Verification items for the finished model (mm, model axes). Give positions to 0.01 mm unless a question says otherwise; leave off trailing zeros. Order: outer loops, then holes, each group sorted by start corner. A loop starts at its lowest first (then second) coordinate and runs counter-clockwise, first axis right, second up. Notation, with made-up numbers: (62.25, 49.25) - (114.25, 49.25) arc R10 ccw to (114.25, 65.25) - close; hole circle Ø3 at (86.25, -34.5). An arc over 180 degrees is marked (long way). Answer as a JSON object with one key per item and string values. Group by question number.
(1) Section check A-A (z = -312). Record the boundary of the cut face in (x, y), then the cut area to 4 significant figures.
(2) Depth check by flat-ended pin: pin 1 Ø2.5 at (y, z) = (2, -197) entering from +X; pin 2 Ø1.5 at (y, z) = (1.5, -390.5) entering from +X; pin 3 Ø1.5 at (x, y) = (-41, 2) entering from -Z. Enter the tip coordinate at first touch or a pass-through.
(3) Section check B-B (y = 3.5). Count the separate pieces of the cut face and the enclosed holes in it, then the cut area to 3 significant figures.
(4) Section check C-C (x = -154). Record the boundary of the cut face in (y, z), then the cut area to 3 significant figures.
(5) Thickness scan on line 1 (Z direction, x = -295, y = 1.35) (1 decimal); line 2 (X direction, y = 4.1, z = -188) (3 decimals); line 3 (X direction, y = 1.9, z = -66.5). Record the ranges inside material, lowest first.
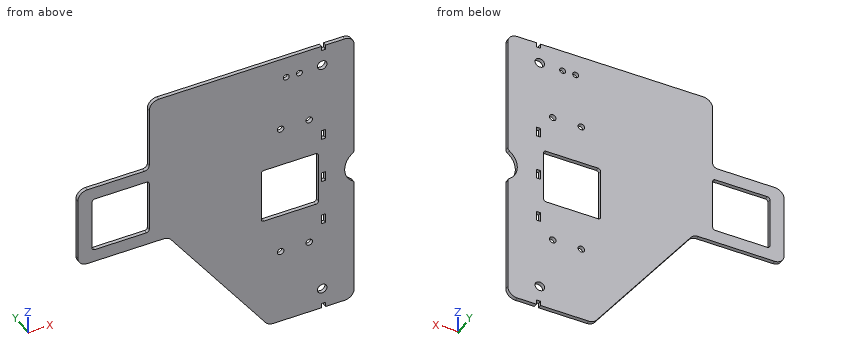
Autodesk Inventor part; units mm, degrees
ref_plane "YZ Plane" through (0, 0, 0) normal (1, 0, 0) x (0, 1, 0)
ref_plane "XZ Plane" through (0, 0, 0) normal (0, 1, 0) x (-1, 0, 0)
ref_plane "XY Plane" through (0, 0, 0) normal (0, 0, 1) x (1, 0, 0)
sketch "Boceto1" plane through (0, 0, 0) normal (0, 1, 0) x (-1, 0, 0)
  line L0 (0, 0) -> (273.05, 0)
  line L1 (273.05, 0) -> (273.05, -101.6)
  line L2 (273.05, -101.6) -> (368.3, -101.6)
  line L3 (368.3, -101.6) -> (368.3, -212.725)
  line L4 (0, 0) -> (0, -393.7)
  line L5 (0, -393.7) -> (114.3, -393.7)
  line L6 (368.3, -212.725) -> (247.65, -212.725)
  line L7 (247.65, -212.725) -> (114.3, -393.7)
  dimension "d0" = 273.05
  dimension "d1" = 101.6
  dimension "d2" = 95.25
  dimension "d3" = 111.125
  dimension "d4" = 393.7
  dimension "d50" = 114.3
  dimension "d51" = 133.35
extrude "Extrusión1" add sketch "Boceto1" along normal blind 5
fillet "Empalme1" radius 12.7 7 edges at (-368.3, 2.5, -101.6) (-273.05, 2.5, 0) (-368.3, 2.5, -212.725) (-247.65, 2.5, -212.725) (-114.3, 2.5, -393.7) (0, 2.5, -393.7) (0, 2.5, 0)
fillet "Empalme2" radius 6.35 1 edges at (-273.05, 2.5, -101.6)
sketch "Boceto2" plane through (0, 5, 0) normal (0, 1, 0) x (1, 0, 0)
  line L0 (-349.25, 119.0625) -> (-273.05, 119.0625)
  line L1 (-273.05, 119.0625) -> (-273.05, 195.2625)
  line L2 (-273.05, 195.2625) -> (-349.25, 195.2625)
  line L3 (-349.25, 195.2625) -> (-349.25, 119.0625)
  line L4 (-368.3, 200.025) -> (-368.3, 114.3)
  line L5 (-254.0674, 212.725) -> (-355.6, 212.725)
  line L6 (-355.6, 101.6) -> (-279.4, 101.6)
  line L7 (-260.35, 0) -> (-12.7, 0)
  line L8 (-43.6563, 0) -> (-38.1, 0)
  line L9 (-38.1, 0) -> (-38.1, 6.35)
  line L10 (-38.1, 6.35) -> (-43.6562, 6.35)
  line L11 (-43.6562, 6.35) -> (-43.6563, 0)
  line L12 (-12.7, 393.7) -> (-107.8826, 393.7)
  line L13 (0, 12.7) -> (0, 381)
  circle A0 centre (-98.0281, 104.775) radius 4.3656
  circle A1 centre (-59.9281, 104.775) radius 4.3656
  circle A2 centre (-98.0281, 288.925) radius 4.3656
  circle A3 centre (-59.9281, 288.925) radius 4.3656
  line L14 (-123.825, 158.75) -> (-47.625, 158.75)
  line L15 (-47.625, 158.75) -> (-47.625, 234.95)
  line L16 (-47.625, 234.95) -> (-123.825, 234.95)
  line L17 (-123.825, 234.95) -> (-123.825, 158.75)
  circle A4 centre (-42.6641, 365.125) radius 6.35
  circle A5 centre (-42.6641, 28.575) radius 6.35
  line L18 (-107.8826, 393.7) -> (-12.7, 393.7)
  line L19 (-43.6563, 393.7) -> (-38.1, 393.7)
  line L20 (-38.1, 393.7) -> (-38.1, 387.35)
  line L21 (-38.1, 387.35) -> (-43.6563, 387.35)
  line L22 (-43.6563, 387.35) -> (-43.6563, 393.7)
  line L23 (-43.6563, 127) -> (-38.1, 127)
  line L24 (-38.1, 127) -> (-38.1, 140.0969)
  line L25 (-38.1, 140.0969) -> (-43.6563, 140.0969)
  line L26 (-43.6563, 140.0969) -> (-43.6563, 127)
  line L27 (-43.6563, 190.5) -> (-38.1, 190.5)
  line L28 (-38.1, 190.5) -> (-38.1, 203.5969)
  line L29 (-38.1, 203.5969) -> (-43.6563, 203.5969)
  line L30 (-43.6563, 203.5969) -> (-43.6563, 190.5)
  line L31 (-43.6563, 254) -> (-38.1, 254)
  line L32 (-38.1, 254) -> (-38.1, 267.0969)
  line L33 (-38.1, 267.0969) -> (-43.6563, 267.0969)
  line L34 (-43.6563, 267.0969) -> (-43.6563, 254)
  circle A6 centre (-73.025, 29.3688) radius 3.9687
  circle A7 centre (-90.4875, 29.3688) radius 3.9688
  point P0 (0, 0)
  dimension "d11" = 76.2
  dimension "d17" = 17.4625
  dimension "d18" = 19.05
  dimension "d19" = 76.2
  dimension "d20" = 5.5563
  dimension "d22" = 6.35
  dimension "d24" = 38.1
  dimension "d27" = 8.7312
  dimension "d38" = 76.2
  dimension "d39" = 76.2
  dimension "d40" = 158.75
  dimension "d42" = 12.7
  dimension "d43" = 28.575
  dimension "d44" = 42.6641
  dimension "d47" = 12.7
  dimension "d52" = 38.1
  dimension "d53" = 5.5563
  dimension "d54" = 6.35
  dimension "d55" = 47.625
  dimension "d56" = 8.7312
  dimension "d57" = 98.0281
  dimension "d58" = 38.1
  dimension "d59" = 53.975
  dimension "d60" = 53.975
  dimension "d61" = 184.15
  dimension "d62" = 184.15
  dimension "d63" = 38.1
  dimension "d64" = 8.7312
  dimension "d65" = 8.7312
  dimension "d66" = 98.0281
  dimension "d67" = 42.6641
  dimension "d68" = 28.575
  dimension "d69" = 5.5563
  dimension "d70" = 5.5563
  dimension "d71" = 5.5563
  dimension "d72" = 13.0969
  dimension "d73" = 13.0969
  dimension "d74" = 13.0969
  dimension "d75" = 38.1
  dimension "d80" = 63.5
  dimension "d81" = 63.5
  dimension "d82" = 127
  dimension "d92" = 7.9375
  dimension "d93" = 7.9375
  dimension "d94" = 25.4
  dimension "d96" = 25.4
  dimension "d97" = 25.4
  dimension "d98" = 25.4
extrude "Extrusión2" cut sketch "Boceto2" against normal up to next
fillet "Empalme3" radius 3.5719 8 edges at (-349.25, 2.5, -119.0625) (-123.825, 2.5, -158.75) (-349.25, 2.5, -195.2625) (-123.825, 2.5, -234.95) (-273.05, 2.5, -195.2625) (-47.625, 2.5, -234.95) (-273.05, 2.5, -119.0625) (-47.625, 2.5, -158.75)
sketch "Boceto3" plane through (0, 5, 0) normal (0, 1, 0) x (1, 0, 0)
  line L0 (0, 12.7) -> (0, 381)
  line L1 (0, 381) -> (0, 12.7)
  line L2 (0, 196.85) -> (-12.7, 196.85)
  line L3 (0, 196.85) -> (0, 219.075)
  line L4 (0, 196.85) -> (0, 174.625)
  arc A0 (0, 219.075) -> (0, 174.625) centre (13.0969, 196.85) ccw
  point P0 (0, 0)
  dimension "d86" = 12.7
  dimension "d87" = 22.225
  dimension "d88" = 22.225
extrude "Extrusión3" cut sketch "Boceto3" against normal up to next
fillet "Empalme4" radius 4.7625 2 edges at (0, 2.5, -219.075) (0, 2.5, -174.625)
equation "\"d42\" = UBD"
equation "\"d47\" = UBD"
equation "\"LM\" = 76.2"
equation "\"UBD\" = 12.7"
properties part number "CAR SIDE PLATE I"
Solutions:
{
 "1": {"outline": "(-174.5, 0) - (0, 0) - (0, 5) - (-174.5, 5) - close", "area": "872.5 mm2"},
 "2": {"pin 1": "stops at x = -12.66", "pin 2": "stops at x = -3.5", "pin 3": "stops at z = -387.35"},
 "3": {"separate pieces": "1", "enclosed holes": "13", "area": "88,400 mm2"},
 "4": {"outline": "(0, -339.82) - (5, -339.82) - (5, 0) - (0, 0) - close", "area": "1,700 mm2"},
 "5": {"line 1": "z = -212.7 to -195.3, -119.1 to -101.6", "line 2": "x = -368.3 to -349.25, -273.05 to -123.825, -47.625 to -11.134", "line 3": "x = -273.05 to 0"}
}
